```python
from build123d import *

# Parameters (mm, degrees)
SKETCH1_W           = 30
SKETCH1_H           = 30
SKETCH1_R           = 6
BOSS_EXTRUDE1_DEPTH = 12
FILLET1_R           = 2
SKETCH2_R           = 1.5
CUT_EXTRUDE1_DEPTH  = 5


with BuildPart() as part:
    # Sketch1 → Boss-Extrude1 (new body)
    with BuildSketch(Plane(origin=(0, 0, 0), x_dir=(1, 0, 0), z_dir=(0, 1, 0))):
        with Locations((15, 15)):
            Rectangle(SKETCH1_W, SKETCH1_H)
        with Locations(Location((15, 15, 0), (0, 0, 270))):
            Circle(SKETCH1_R, mode=Mode.SUBTRACT)
    extrude(amount=BOSS_EXTRUDE1_DEPTH)

    # Fillet1
    fillet1_edges = [part.edges().sort_by_distance(p)[0] for p in [
        (0, 6, -30),
        (30, 6, -30),
    ]]
    fillet(fillet1_edges, radius=FILLET1_R)

    # Sketch2 → Cut-Extrude1 (cut)
    with BuildSketch(Plane.XY):
        with Locations((5, 6)):
            Circle(SKETCH2_R)
        with Locations(Location((25, 6, 0), (0, 0, 180))):
            Circle(SKETCH2_R)
    extrude(amount=-CUT_EXTRUDE1_DEPTH, mode=Mode.SUBTRACT)


solid = part.part
```
Here's how the part is built. I have some questions about the finished solid (model axes, mm). A direction names the side the tool comes from. Give positions to 0.01 mm unless a question says otherwise; leave off trailing zeros. Loops run counter-clockwise (first coordinate to the right, second up) from the corner with the lowest first, then second, coordinate; pieces in that order, holes last. Notation, with made-up numbers: (24.25, -29.5) -> (66.25, -29.5) arc R29 cw to (66.25, 9.5) -> close; hole circle Ø10 at (55, -26.5). An arc over 180 degrees is marked (long way). Use one line per item in the form item = value. Start each with the question number.
1) Imagine slicing it at B-B (z = -15). Please give me the cut outline in (x, y).
2) Imagine slicing it at C-C (x = 5). Please give me the cut outline in (y, z).
3) Which directions (+Z, -Z, +X, -X, +Y, -Y) give clear straight access to the entire face, cutting with the end or side of a thin tool? Please do faces 5 (the face through (15, 6, -30)), 6 (the face through (26.5, 5.93, -2.46)).
4) Thinking about a two-plate mould opening in Y: for faces 1 (the face through (8, 0, -15)), 2 (the face through (5, 6, -5)), 3 (the face through (8, 12, -15)), 4 (the face through (29.4, 6.08, -29.43)), which applies, +Y half, -Y half, draft (parallel to the pull), parting line (faces both ways), or undercut?
5) Imagine slicing it at A-A (x = 15). Please give me the cut outline in (y, z), then the cut area to 3 significant figures.
6) For P1, Ø3.5, axis at x = 5, y = 6, coming from the +Z side; P2, Ø0.9, axis at x = 24.5, y = 5.5, coming from the +Z side, each with a flat end and sliding along its axis, tell me the tip position at first contact or that it passes through.
7) Imagine slicing it at D-D (y = 6.5). Please give me the cut outline in (x, z).
8) Please list where these lines run through material, in increasing order: line 1 along Y through (x, z) = (25, -2.85); line 2 along X through (y, z) = (6.75, -15); line 3 along Z through (x, y) = (17, 11.5).
Check values:
q1.outline = (0, 0) -> (9, 0) -> (9, 12) -> (0, 12) -> close; (21, 0) -> (30, 0) -> (30, 12) -> (21, 12) -> close
q2.outline = (0, -30) -> (12, -30) -> (12, 0) -> (7.5, 0) -> (7.5, -5) -> (4.5, -5) -> (4.5, 0) -> (0, 0) -> close
q3.face_5 = -Z, +X, -X, +Y, -Y
q3.face_6 = +Z
q4.face_1 = -Y half
q4.face_2 = undercut
q4.face_3 = +Y half
q4.face_4 = draft
q5.outline = (0, -30) -> (12, -30) -> (12, -21) -> (0, -21) -> close; (0, -9) -> (12, -9) -> (12, 0) -> (0, 0) -> close
q5.area = 216 mm^2
q6.P1 = 0
q6.P2 = -5
q7.outline = (0, -28) arc R2 ccw to (2, -30) -> (28, -30) arc R2 ccw to (30, -28) -> (30, 0) -> (26.41, 0) -> (26.41, -5) -> (23.59, -5) -> (23.59, 0) -> (6.41, 0) -> (6.41, -5) -> (3.59, -5) -> (3.59, 0) -> (0, 0) -> close; hole circle Ø12 at (15, -15)
q8.line_1 = 0 to 4.5, 7.5 to 12
q8.line_2 = 0 to 9, 21 to 30
q8.line_3 = -30 to -20.66, -9.34 to 0
